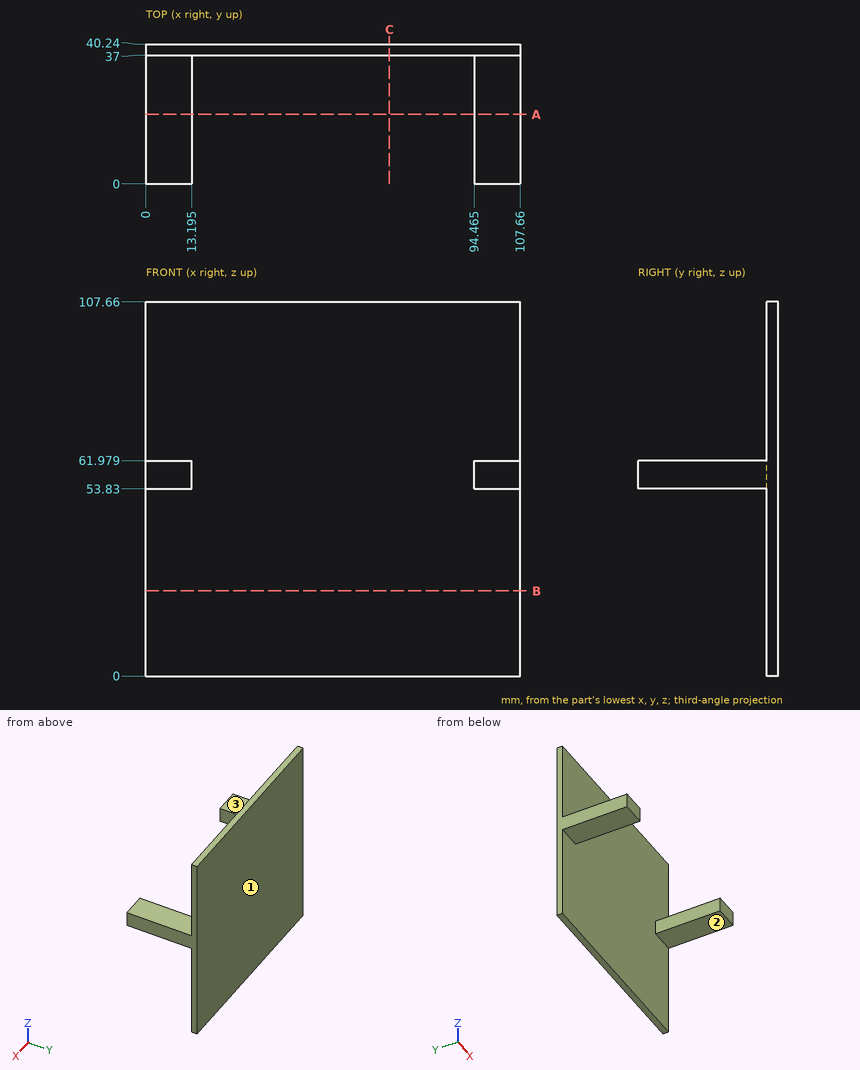
Check sheet for the drawn part. Datum: minimum x, y, z corner. Units: mm. A direction names the side the tool comes from. Round coordinates to 2 decimals unless told otherwise and drop trailing zeros. Order: outer loops, then holes, each group sorted by start corner. A loop starts at its lowest first (then second) coordinate and runs counter-clockwise, first axis right, second up. Notation, with made-up numbers: M 29.5,34 L 58.5,34 A25 ccw 58.5,52 Z; hole C 3.5,39 d1. An arc over 180 degrees is marked long. Write each question's results on one line, items separated by ' | '. Start each with the question number.
1. Cross-section at C-C on x = 70. Record the boundary of the cut face in (y, z).
2. Material ranges on L1, parallel to X at y = 3.5, z = 57.5 (1 decimal); L2, parallel to Y at x = 39.5, z = 49; L3, parallel to Z at x = 9.5, y = 5, recorded low to high. Write a range as from..to.
3. Cross-section at B-B on z = 24.5. Record the boundary of the cut face in (x, y), plus the area to 3 significant figures.
4. Go/stop test with flat-tipped pins: P1, Ø6.5, axis at x = 5.5, y = 18, coming from the +Z side; P2, Ø6, axis at x = 75, y = 32, coming from the -Z side; P3, Ø14.5, axis at x = 102, y = 20, coming from the -Z side; P4, Ø3, axis at x = 20.5, z = 28, coming from the -Y side. Record where each tip stops, or that it passes through.
5. Set-up check for the marked faces 1, 2 and 3: record each of +Z, -Z, +X, -X, +Y, -Y from which the full face is reachable in a straight line by a thin tool's end or side.
6. Cross-section at A-A on y = 20. Record the boundary of the cut face in (x, z) (1 decimal).
Resolved:
1) outline: M 37,0 L 40.24,0 L 40.24,107.66 L 37,107.66 Z
2) L1: 0..13.2, 94.5..107.7 | L2: 37..40.24 | L3: 53.83..61.98
3) outline: M 0,37 L 107.66,37 L 107.66,40.24 L 0,40.24 Z | area: 349 mm2
4) P1: z = 61.98 | P2: through | P3: z = 53.83 | P4: y = 37
5) face 1: +Z, -Z, +X, -X, +Y | face 2: -Z, +X, -X, -Y | face 3: +Z, +X, -X, -Y
6) outline: M 0,53.8 L 13.2,53.8 L 13.2,62 L 0,62 Z; M 94.5,53.8 L 107.7,53.8 L 107.7,62 L 94.5,62 Z
